Input: part model. Units: mm. Frame: model coordinates. Face numbers are marked on the shaded views. Round coordinates to 2 decimals unless told otherwise and drop trailing zeros. Order: outer loops, then holes, each group sorted by start corner. A loop starts at its lowest first (then second) coordinate and runs counter-clockwise, first axis right, second up. Notation, with made-up numbers: (52, -21) -> (62, -21) arc R26 ccw to (62, -7) -> close; hole circle Ø8 at (17.25, 74.25). An arc over 180 degrees is marked (long way). Use a Markdown table: item, result.
Autodesk Inventor part; units mm, degrees
ref_plane "YZ Plane" through (0, 0, 0) normal (1, 0, 0) x (0, 1, 0)
ref_plane "XZ Plane" through (0, 0, 0) normal (0, 1, 0) x (-1, 0, 0)
ref_plane "XY Plane" through (0, 0, 0) normal (0, 0, 1) x (1, 0, 0)
sketch "Эскиз1" plane through (0, 0, 0) normal (0, 0, 1) x (1, 0, 0)
  line L0 (11, 0.5) -> (-11, 0.5)
  line L1 (-11, 0.5) -> (-11, -0.5)
  line L2 (-11, -0.5) -> (11, -0.5)
  line L3 (11, -0.5) -> (11, 0.5)
  line L4 (11, 0.5) -> (-11, -0.5) construction
  line L5 (-11, 0.5) -> (11, -0.5) construction
  line L6 (-11, 2) -> (11, 2)
  line L7 (11, 2) -> (11, 3)
  line L8 (11, 3) -> (-11, 3)
  line L9 (-11, 3) -> (-11, 2)
  line L10 (-11, 4.5) -> (11, 4.5)
  line L11 (11, 4.5) -> (11, 5.5)
  line L12 (11, 5.5) -> (-11, 5.5)
  line L13 (-11, 5.5) -> (-11, 4.5)
  line L14 (-11, 7) -> (11, 7)
  line L15 (11, 7) -> (11, 8)
  line L16 (11, 8) -> (-11, 8)
  line L17 (-11, 8) -> (-11, 7)
  line L18 (-11, 9.5) -> (11, 9.5)
  line L19 (11, 9.5) -> (11, 10.5)
  line L20 (11, 10.5) -> (-11, 10.5)
  line L21 (-11, 10.5) -> (-11, 9.5)
  line L22 (-11, 12) -> (11, 12)
  line L23 (11, 12) -> (11, 13)
  line L24 (11, 13) -> (-11, 13)
  line L25 (-11, 13) -> (-11, 12)
  line L26 (-11, 14.5) -> (11, 14.5)
  line L27 (11, 14.5) -> (11, 15.5)
  line L28 (11, 15.5) -> (-11, 15.5)
  line L29 (-11, 15.5) -> (-11, 14.5)
  line L30 (-11, 17) -> (11, 17)
  line L31 (11, 17) -> (11, 18)
  line L32 (11, 18) -> (-11, 18)
  line L33 (-11, 18) -> (-11, 17)
  line L34 (-11, 19.5) -> (11, 19.5)
  line L35 (11, 19.5) -> (11, 20.5)
  line L36 (11, 20.5) -> (-11, 20.5)
  line L37 (-11, 20.5) -> (-11, 19.5)
  line L38 (-11, 22) -> (11, 22)
  line L39 (11, 22) -> (11, 23)
  line L40 (11, 23) -> (-11, 23)
  line L41 (-11, 23) -> (-11, 22)
  line L42 (-11, 24.5) -> (11, 24.5)
  line L43 (11, 24.5) -> (11, 25.5)
  line L44 (11, 25.5) -> (-11, 25.5)
  line L45 (-11, 25.5) -> (-11, 24.5)
  line L46 (0, -0.5) -> (0, 25.5)
  circle A0 centre (0, 24.5) radius 4.8 construction
  circle A1 centre (0, 0.5) radius 6 construction
  line L47 (-6, 0.5) -> (-4.8, 24.5)
  line L48 (6, 0.5) -> (4.8, 24.5)
  point P0 (0, 0)
  point P1 (0, 0)
  point P2 (0, 2)
  point P3 (0, 3)
  point P4 (0, 4.5)
  point P5 (0, 7)
  point P6 (0, 5.5)
  point P7 (0, 9.5)
  point P8 (0, 8)
  point P9 (0, 12)
  point P10 (0, 10.5)
  point P11 (0, 14.5)
  point P12 (0, 13)
  point P13 (0, 17)
  point P14 (0, 15.5)
  point P15 (0, 18)
  point P16 (0, 19.5)
  point P17 (0, 22)
  point P18 (0, 20.5)
  point P19 (-4.925, 22)
  point P20 (-4.875, 23)
  point P21 (-5.125, 18)
  point P22 (-5.175, 17)
  point P23 (-5.25, 15.5)
  point P24 (-5.3, 14.5)
  point P25 (-5.375, 13)
  point P26 (-5.425, 12)
  point P27 (-5.5, 10.5)
  point P28 (0, 9.5)
  point P29 (0, 22)
  point P30 (0, 23)
  point P31 (-5.675, 7)
  point P32 (-5.625, 8)
  point P33 (-5.8, 4.5)
  point P34 (-5.75, 5.5)
  point P35 (-5.875, 3)
  point P36 (-5.925, 2)
  point P37 (0, 4.5)
  point P38 (0, 5.5)
  point P39 (0, 7)
  point P40 (-5.55, 9.5)
  point P41 (0, 8)
  point P42 (-5.05, 19.5)
  point P43 (-5, 20.5)
  dimension "d0" = 22
  dimension "d1" = 1
  dimension "d2" = 1.5
  dimension "d3" = 1.5
  dimension "d4" = 1.5
  dimension "d5" = 1.5
  dimension "d6" = 1.5
  dimension "d7" = 1.5
  dimension "d8" = 1.5
  dimension "d9" = 1.5
  dimension "d10" = 1.5
  dimension "d11" = 1
  dimension "d12" = 1
  dimension "d13" = 1
  dimension "d14" = 1
  dimension "d15" = 1
  dimension "d16" = 1
  dimension "d17" = 1
  dimension "d18" = 1
  dimension "d19" = 1
  dimension "d20" = 1
  dimension "d21" = 1.5
  dimension "d22" = 9.6
  dimension "d23" = 12
revolve "Вращение1" add sketch "Эскиз1" angle 360 about axis through (0, -0.5, 0) along (0, 1, 0) contours L46 L2 L1 L0 | L0 L47 L6 L46 | L6 L47 L8 L46 | L6 L9 L8 L47 | L8 L47 L10 L46 | L10 L47 L12 L46 | L10 L13 L12 L47 | L12 L47 L14 L46 | L14 L47 L16 L46 | L14 L17 L16 L47 | L16 L47 L18 L46 | L18 L47 L20 L46 | L18 L21 L20 L47 | L20 L47 L22 L46 | L22 L47 L24 L46 | L22 L25 L24 L47 | L24 L47 L26 L46 | L26 L47 L28 L46 | L26 L29 L28 L47 | L28 L47 L30 L46 | L30 L47 L32 L46 | L30 L33 L32 L47 | L32 L47 L34 L46 | L34 L47 L36 L46 | L34 L37 L36 L47 | L36 L47 L38 L46 | L38 L47 L40 L46 | L38 L41 L40 L47 | L40 L47 L42 L46 | L42 L45 L44 L46
sketch "Эскиз2" plane through (0, -0.5, 0) normal (0, -1, 0) x (1, 0, 0)
  circle A0 centre (0, 0) radius 3.5
  dimension "d25" = 7
extrude "Выдавливание1" cut sketch "Эскиз2" against normal blind 12
sketch "Эскиз3" plane through (0, 25.5, 0) normal (0, 1, 0) x (1, 0, 0)
  circle A0 centre (0, 0) radius 2.1
  dimension "d28" = 4.2
extrude "Выдавливание2" cut sketch "Эскиз3" against normal through all
sketch "Эскиз4" plane through (0, 25.5, 0) normal (0, 1, 0) x (1, 0, 0)
  circle A0 centre (0, 0) radius 8 construction
  circle A1 centre (0, 8) radius 1.25
  circle A2 centre (-8, 0) radius 1.25
  circle A3 centre (0, -8) radius 1.25
  circle A4 centre (8, 0) radius 1.25
  dimension "d31" = 16
  dimension "d32" = 2.5
  dimension "d35" = 360
extrude "Выдавливание3" cut sketch "Эскиз4" against normal up to surface (3.5 mm away)
chamfer "Фаска1" distance 0.5 angle 45 1 edges at (-3.5, -0.5, 0)
properties part number "Radiator"
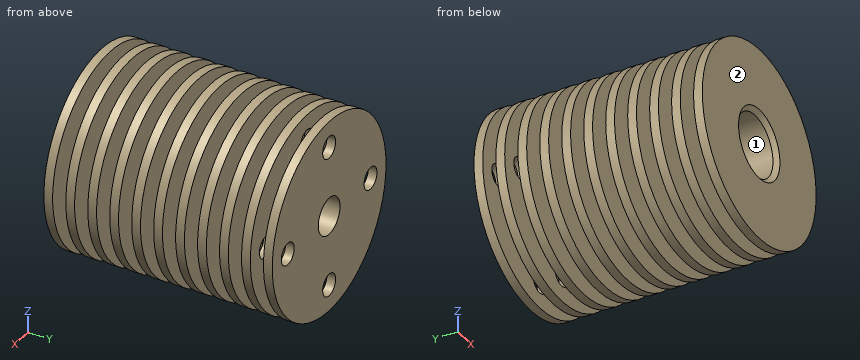
1) Pin query (flat end, axial travel): pin 1 Ø11 at (x, z) = (-1, -1.5) entering from -Y; pin 2 Ø5 at (x, y) = (8.5, 5) entering from -Z; pin 3 Ø4 at (x, y) = (5, 21) entering from -Z; pin 4 Ø2 at (x, y) = (1.5, 7.5) entering from +Z. Return the tip coordinate at first contact, or that it passes through.
Results found:
| item | result |
|---|---|
| pin 1 | stops at y = -0.5 |
| pin 2 | stops at z = -9.22 |
| pin 3 | stops at z = -10.56 |
| pin 4 | stops at z = 10.99 |
2) Line query: L1, parallel to Z at x = 0, y = 22.6; L2, parallel to Z at x = -8, y = 22.85; L3, parallel to X at y = 22.75, z = -7. Output: solid intervals per line, ascending. Write a range as [from, to].
Results found:
| item | result |
|---|---|
| L1 | z = [-11, -9.25], [-6.75, -2.1], [2.1, 6.75], [9.25, 11] |
| L2 | z = [-7.55, -1.25], [1.25, 7.55] |
| L3 | x = [-8.49, -0.75], [0.75, 8.49] |
3) Cut plane B-B on z = 0. Count the separate pieces of the cut face and the enclosed holes in it, and give its area (3 significant figures).
Results found:
| item | result |
|---|---|
| separate pieces | 6 |
| enclosed holes | 0 |
| area | 251 mm² |
4) Pull-direction query (Z, two-part tool) for the marked faces 1 and 2; classes: +Z half, -Z half, draft (parallel to the pull), parting line (faces both ways), or undercut.
Results found:
| item | result |
|---|---|
| face 1 | undercut |
| face 2 | draft |
5) Cut plane A-A on y = 10. Return loops of the section in (x, z).
Results found:
| item | result |
|---|---|
| outline | circle Ø22 at (0, 0); hole circle Ø7 at (0, 0) |
